CAD build for the part. Positions are in the model's coordinates, mm. Face numbers are marked on the shaded views. A direction names the side the tool comes from. Round coordinates to 2 decimals unless told otherwise and drop trailing zeros. Write each loop counter-clockwise with the first axis right and the second up, starting at its lowest first coordinate (ties: lowest second). Pieces come first, ordered by that corner, then holes. Notation, with made-up numbers: (30.5, 4) - (45.5, 4) arc R12 cw to (45.5, 23) - close; hole circle Ø9 at (68.25, 64). An arc over 180 degrees is marked (long way). Use one line per item in the form item = value. Start each with the question number.
Item 1: Band-saw the part on C-C, the plane z = 2. List the corners of the cut face in (x, y), and give its area (3 significant figures).
Item 2: Pull direction Y, two halves, no side cores. Call the marked faces 3, 4 and 5: +Y half, -Y half, draft (parallel to the pull), parting line (faces both ways), or undercut.
Item 3: Tool access for the marked faces 1 and 2: list every direction of +Z, -Z, +X, -X, +Y, -Y with a clear straight run to the whole face (end or side of a thin tool).
Item 4: Band-saw the part on D-D, the plane y = 35. List the corners of the cut face in (x, z).
Item 5: Band-saw the part on B-B, the plane y = 0. List the corners of the cut face in (x, z).
Item 6: Drill centre lines: L1, parallel to Y at x = 0, z = -4.25; L2, parallel to Z at x = -7, y = -35.5; L3, parallel to X at y = 35, z = 1.85. Where is each one in solid material? Low to high.
Item 7: Pin check, flat tips, straight feed: pin 1 (6 mm diameter, centred on x = 25, z = 0, fed in from -Y); pin 2 (4 mm diameter, centred on x = -16, z = -6, fed in from +Y); pin 3 (2.5 mm diameter, centred on x = 25, y = 0, fed in from -Z); pin 4 (8 mm diameter, centred on x = 0.5, z = 1.5, fed in from +Y). Stop position of each tip, or through.
Item 8: Band-saw the part on A-A, the plane x = 0. List the corners of the cut face in (y, z).
from build123d import *

# Parameters (mm, degrees)
CROQUIS1_R              = 40
SALIENTE_EXTRUIR1_DEPTH = 5
CROQUIS3_R              = 27.5
SALIENTE_EXTRUIR2_DEPTH = 10
TALADRO_ROSCADO_M41_D   = 3.3
CROQUIS6_R              = 10.25
CORTAR_EXTRUIR1_DEPTH   = 34.8


with BuildPart() as part:
    # Croquis1 → Saliente-Extruir1 (new body)
    with BuildSketch(Plane.XY):
        Circle(CROQUIS1_R)
    extrude(amount=SALIENTE_EXTRUIR1_DEPTH)

    # Croquis2 → Cortar-Revolución1 (revolve, cut)
    with BuildSketch(Plane(origin=(0, 0, 0), x_dir=(0, 0, -1), z_dir=(1, 0, 0))):
        Polygon((-5, 35), (-5, 39), (-3.2, 37.25), (0, 37.25), (0, 35), align=None)
    revolve(axis=Axis((0, 35, 20.622839442), (0, 0, -1)), mode=Mode.SUBTRACT)

    # Croquis3 → Saliente-Extruir2 (add)
    with BuildSketch(Plane(origin=(0, 0, 0), x_dir=(-1, 0, 0), z_dir=(0, 0, -1))):
        Circle(CROQUIS3_R)
    extrude(amount=SALIENTE_EXTRUIR2_DEPTH)

    # Taladro roscado M41 (through all)
    with Locations(Plane.XY.offset(5)):
        with Locations((-25, 0), (25, 0)):
            Hole(TALADRO_ROSCADO_M41_D / 2)

    # Croquis6 → Cortar-Extruir1 (cut)
    with BuildSketch(Plane.XY.offset(5)):
        Circle(CROQUIS6_R)
    extrude(amount=-CORTAR_EXTRUIR1_DEPTH, mode=Mode.SUBTRACT)


solid = part.part
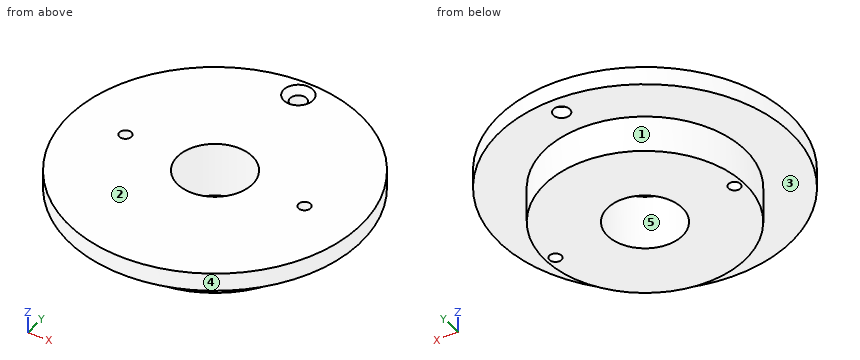
Determined:
q1.outline = circle Ø80 at (0, 0); hole circle Ø3.3 at (-25, 0); hole circle Ø20.5 at (0, 0); hole circle Ø4.5 at (0, 35); hole circle Ø3.3 at (25, 0)
q1.area = 4,660 mm²
q2.face_3 = draft
q2.face_4 = parting line
q2.face_5 = undercut
q3.face_1 = -Z
q3.face_2 = +Z, +X, -X, +Y, -Y
q4.outline = (-19.36, 0) - (-2.25, 0) - (-2.25, 3.2) - (-4, 5) - (-19.36, 5) - close; (2.25, 0) - (19.36, 0) - (19.36, 5) - (4, 5) - (2.25, 3.2) - close
q5.outline = (-40, 0) - (-27.5, 0) - (-27.5, -10) - (-26.65, -10) - (-26.65, 5) - (-40, 5) - close; (-23.35, -10) - (-10.25, -10) - (-10.25, 5) - (-23.35, 5) - close; (10.25, -10) - (23.35, -10) - (23.35, 5) - (10.25, 5) - close; (26.65, -10) - (27.5, -10) - (27.5, 0) - (40, 0) - (40, 5) - (26.65, 5) - close
q6.L1 = -27.5 to -10.25, 10.25 to 27.5
q6.L2 = 0 to 5
q6.L3 = -19.36 to -2.25, 2.25 to 19.36
q7.pin_1 = -33.41
q7.pin_2 = 23.67
q7.pin_3 = through
q7.pin_4 = 40
q8.outline = (-40, 0) - (-27.5, 0) - (-27.5, -10) - (-10.25, -10) - (-10.25, 5) - (-40, 5) - close; (10.25, -10) - (27.5, -10) - (27.5, 0) - (32.75, 0) - (32.75, 3.2) - (31, 5) - (10.25, 5) - close; (37.25, 0) - (40, 0) - (40, 5) - (39, 5) - (37.25, 3.2) - close
